Model file for the job. Use its own axes, mm. A direction names the side the tool comes from. Give positions to 0.01 mm unless a question says otherwise; leave off trailing zeros. Write each loop counter-clockwise with the first axis right and the second up, starting at its lowest first coordinate (ties: lowest second). Pieces come first, ordered by that corner, then holes.
```python
from build123d import *

# Parameters (mm, degrees)
SKETCH1_W               = 14.07
SKETCH1_H               = 24
BOSS_EXTRUDE1_DEPTH     = 24.27
SKETCH3_W               = 12.07
SKETCH3_H               = 22
CUT_EXTRUDE1_DEPTH      = 23.27
CUT_EXTRUDE2_DEPTH      = 37.918800089
CUT_EXTRUDE2_DEPTH_BACK = 37.918800089
SKETCH5_W               = 12.07
SKETCH5_H               = 3.69525946
SKETCH6_W               = 10
SKETCH6_H               = 10
BOSS_EXTRUDE2_DEPTH     = 27
SKETCH7_W               = 4.035
SKETCH7_H               = 10
BOSS_EXTRUDE3_DEPTH     = 80


with BuildPart() as part:
    # Sketch1 → Boss-Extrude1 (new body)
    with BuildSketch(Plane(origin=(0, 0, 0), x_dir=(1, 0, 0), z_dir=(0, 1, 0))):
        with Locations((7.035, 12)):
            Rectangle(SKETCH1_W, SKETCH1_H)
    extrude(amount=BOSS_EXTRUDE1_DEPTH)

    # Sketch3 → Cut-Extrude1 (cut)
    with BuildSketch(Plane(origin=(0, 24.27, 0), x_dir=(1, 0, 0), z_dir=(0, 1, 0))):
        with Locations((7.035, 12)):
            Rectangle(SKETCH3_W, SKETCH3_H)
    extrude(amount=-CUT_EXTRUDE1_DEPTH, mode=Mode.SUBTRACT)

    # Sketch5 → Cut-Extrude2 (cut, two sides: drawn at the far end of the back side and taken through both)
    with BuildSketch(Plane(origin=(0, 0, -24), x_dir=(-1, 0, 0), z_dir=(0, 0, -1)).offset(-CUT_EXTRUDE2_DEPTH_BACK)):
        with Locations((-7.035, 19.31762973)):
            Rectangle(SKETCH5_W, SKETCH5_H)
    extrude(amount=CUT_EXTRUDE2_DEPTH + CUT_EXTRUDE2_DEPTH_BACK, mode=Mode.SUBTRACT)

    # Sketch6 → Boss-Extrude2 (add)
    with BuildSketch(Plane(origin=(14.07, 0, 0), x_dir=(0, 0, -1), z_dir=(1, 0, 0))):
        with Locations((19, 5)):
            Rectangle(SKETCH6_W, SKETCH6_H)
    extrude(amount=BOSS_EXTRUDE2_DEPTH)

    # Sketch7 → Boss-Extrude3 (add)
    with BuildSketch(Plane.XY.offset(-14)):
        with Locations((39.0525, 5)):
            Rectangle(SKETCH7_W, SKETCH7_H)
    extrude(amount=BOSS_EXTRUDE3_DEPTH)


solid = part.part
```
1. Slice it at D-D, the plane y = 4.25. Write the cut outline in (x, z) (3 decimals).
Calculated:
outline: (0, -24) - (41.07, -24) - (41.07, 66) - (37.035, 66) - (37.035, -14) - (14.07, -14) - (14.07, 0) - (0, 0) - close; hole (1, -23) - (13.07, -23) - (13.07, -1) - (1, -1) - close
2. Slice it at C-C, the plane x = 6. Write the cut outline in (y, z).
Calculated:
outline: (0, -24) - (17.47, -24) - (17.47, -23) - (1, -23) - (1, -1) - (17.47, -1) - (17.47, 0) - (0, 0) - close; (21.17, -24) - (24.27, -24) - (24.27, -23) - (21.17, -23) - close; (21.17, -1) - (24.27, -1) - (24.27, 0) - (21.17, 0) - close
3. Which spindle directions (+Z, -Z, +X, -X, +Y, -Y) get a long thin tool onto all of the face, cutting with end or side? Do faces 4 (the flat face through (7, 1, -12)), 5 (the flat face through (37.035, 5, 25)), 6 (the flat face through (7, 12, 0)), 7 (the flat face through (14.07, 15, -9)). Say none if no direction does.
Calculated:
face 4: +Y
face 5: +Z, +Y, -Y
face 6: +Z, -X, +Y, -Y
face 7: +Z, +Y
4. Slice it at A-A, the plane z = -13. Write the cut outline in (x, y) (3 decimals).
Calculated:
outline: (0, 0) - (14.07, 0) - (14.07, 24.27) - (13.07, 24.27) - (13.07, 1) - (1, 1) - (1, 24.27) - (0, 24.27) - close; (37.035, 0) - (41.07, 0) - (41.07, 10) - (37.035, 10) - close
5. Slice it at B-B, the plane y = 18.5. Write the cut outline in (x, z), and give its area (3 significant figures).
Calculated:
outline: (0, -24) - (1, -24) - (1, 0) - (0, 0) - close; (13.07, -24) - (14.07, -24) - (14.07, 0) - (13.07, 0) - close
area: 48.0 mm2
6. Pin check, flat tips, straight feed: P1, Ø8, axis at x = 23, y = 16, coming from the -Z side; P2, Ø2.5, axis at x = 4.5, y = 22.5, coming from the +Z side; P3, Ø1.1, axis at x = 7.5, z = -0.5, coming from the -Y side; P4, Ø5, axis at y = 5, z = 36, coming from the -X side (3 decimals). Stop position of each tip, or through.
Calculated:
P1: passes through
P2: stops at z = 0
P3: stops at y = 0
P4: stops at x = 37.035
7. Pull direction X, two halves, no side cores. Call faces 1 (the flat face through (0, 12, -12)), 2 (the flat face through (7, 9, -1)), 3 (the flat face through (39, 5, 66)): +X half, -X half, draft (parallel to the pull), parting line (faces both ways), or undercut.
Calculated:
face 1: -X half
face 2: undercut
face 3: draft
8. Probe probe 1 along X at (y, z) = (15.5, -4.5); probe 2 along Z at (x, y) = (9, 11.5); probe 3 along X at (y, z) = (9, -1.5) (3 decimals). List the from-to ranges inside material, lowest first.
Calculated:
probe 1: x = 0 to 1, 13.07 to 14.07
probe 2: z = -24 to -23, -1 to 0
probe 3: x = 0 to 1, 13.07 to 14.07, 37.035 to 41.07
